Can you work these out from the model? Positions are in its coordinate system, mm. A direction names the side the tool comes from. Coordinates: 2 decimals unless noted, no trailing zeros. Loops run counter-clockwise (first coordinate to the right, second up) from the corner with the lowest first, then second, coordinate; pieces in that order, holes last.
```python
from build123d import *

# Parameters (mm, degrees)
SKETCH_1_W                  = 35
SKETCH_1_H                  = 42
EXTRUDE_1_DEPTH             = 4
SKETCH_2_R                  = 1.5
SKETCH_2_R_2                = 9
CUT_EXTRUDE_1_DEPTH         = 8
SKETCH_3_R                  = 3
CUT_EXTRUDE_2_DEPTH         = 4
HOLE_WIZARD_M4_1_AT_2_COUNT = 2
HOLE_WIZARD_M4_1_AT_2_PITCH = 25
SKETCH_9_R                  = 2
CUT_EXTRUDE_3_DEPTH         = 5.1
CUT_EXTRUDE_4_DEPTH         = 29.482450737
CUT_EXTRUDE_4_DEPTH_BACK    = 29.482450737
SKETCH_10_W                 = 15
SKETCH_10_H                 = 8
SKETCH_10_W_2               = 5
SKETCH_10_H_2               = 20
FILLET_2_R                  = 1
CHAMFER_1_SIZE              = 1


with BuildPart() as part:
    # 草图1 → 凸台-拉伸1 (new, symmetric)
    with BuildSketch(Plane.XY):
        Rectangle(SKETCH_1_W, SKETCH_1_H)
    extrude(amount=EXTRUDE_1_DEPTH, both=True)

    # 草图2 → 切除-拉伸1 (cut)
    with BuildSketch(Plane.XY.offset(4)):
        with Locations((0, 13.5)):
            Circle(SKETCH_2_R)
        with Locations((11.691342951, -6.75)):
            Circle(SKETCH_2_R)
        with Locations((-11.691342951, -6.75)):
            Circle(SKETCH_2_R)
        Circle(SKETCH_2_R_2)
    extrude(amount=-CUT_EXTRUDE_1_DEPTH, mode=Mode.SUBTRACT)

    # 草图3 → 切除-拉伸2 (cut)
    with BuildSketch(Plane.XY.offset(4)):
        with Locations((-11.691342951, -6.75)):
            Circle(SKETCH_3_R)
        with Locations((11.691342951, -6.75)):
            Circle(SKETCH_3_R)
        with Locations((0, 13.5)):
            Circle(SKETCH_3_R)
    extrude(amount=-CUT_EXTRUDE_2_DEPTH, mode=Mode.SUBTRACT)

    # 草图8 → M4 螺纹孔1 (revolve, cut)
    with BuildSketch(Plane(origin=(-12.5, 21, 0), x_dir=(0, 0, 1), z_dir=(1, 0, 0))):
        Polygon((0, 0), (0, 10.991420021), (1.65, 10), (1.65, 0), align=None)
    hole_wizard_m4_1 = revolve(axis=Axis((-12.5, 27.35, 0), (0, -1, 0)), mode=Mode.SUBTRACT)

    # M4 螺纹孔1 at 2: M4 螺纹孔1 ×2
    with Locations(*[(i * HOLE_WIZARD_M4_1_AT_2_PITCH, 0, 0) for i in range(1, HOLE_WIZARD_M4_1_AT_2_COUNT)]):
        add(hole_wizard_m4_1, mode=Mode.SUBTRACT)

    # 镜向1: M4 螺纹孔1 across plane
    add(hole_wizard_m4_1.mirror(Plane.ZX), mode=Mode.SUBTRACT)

    # 镜向1 copy 1 sketch → 镜向1 copy 1 (revolve, cut)
    with BuildSketch(Plane(origin=(12.5, -21, 0), x_dir=(0, 0, 1), z_dir=(1, 0, 0))):
        Polygon((0, 0), (0, -10.991420021), (1.65, -10), (1.65, 0), align=None)
    revolve(axis=Axis((12.5, -27.35, 0), (0, -1, 0)), mode=Mode.SUBTRACT)

    # 草图9 → 切除-拉伸3 (cut)
    with BuildSketch(Plane(origin=(0, 0, -4), x_dir=(-1, 0, 0), z_dir=(0, 0, -1))):
        with Locations((0, -12.15)):
            Circle(SKETCH_9_R)
        with Locations((-10.522208656, 6.075)):
            Circle(SKETCH_9_R)
        with Locations((10.522208656, 6.075)):
            Circle(SKETCH_9_R)
    extrude(amount=-CUT_EXTRUDE_3_DEPTH, mode=Mode.SUBTRACT)

    # 草图10 → 切除-拉伸4 (cut, two sides: drawn at the far end of the back side and taken through both)
    with BuildSketch(Plane(origin=(0, 0, -4), x_dir=(-1, 0, 0), z_dir=(0, 0, -1)).offset(-CUT_EXTRUDE_4_DEPTH_BACK)):
        with Locations((0, 21)):
            Rectangle(SKETCH_10_W, SKETCH_10_H)
        with Locations((0, -21)):
            Rectangle(SKETCH_10_W, SKETCH_10_H)
        with Locations((17.5, 0)):
            Rectangle(SKETCH_10_W_2, SKETCH_10_H_2)
        with Locations((-17.5, 0)):
            Rectangle(SKETCH_10_W_2, SKETCH_10_H_2)
    extrude(amount=CUT_EXTRUDE_4_DEPTH + CUT_EXTRUDE_4_DEPTH_BACK, mode=Mode.SUBTRACT)

    # 圆角2
    fillet_2_edges = [part.edges().sort_by_distance(p)[0] for p in [
        (-7.5, 21, 0),
        (-7.5, 17, 0),
        (7.5, 21, 0),
        (7.5, 17, 0),
        (-7.5, -21, 0),
        (-7.5, -17, 0),
        (7.5, -21, 0),
        (7.5, -17, 0),
        (-17.5, -10, 0),
        (-15, -10, 0),
        (-17.5, 10, 0),
        (-15, 10, 0),
        (15, 10, 0),
        (17.5, -10, 0),
        (15, -10, 0),
        (17.5, 10, 0),
        (17.5, -21, 0),
        (-17.5, -21, 0),
        (-17.5, 21, 0),
        (17.5, 21, 0),
    ]]
    fillet(fillet_2_edges, radius=FILLET_2_R)

    # 倒角1
    chamfer_1_edges = [part.edges().sort_by_distance(p)[0] for p in [
        (-9, 0, -4),
        (-9, 0, 4),
    ]]
    chamfer(chamfer_1_edges, length=CHAMFER_1_SIZE)


solid = part.part
```
Item 1: We'd pull the mould along Y, two halves only. Please class faces 4 (the face through (-14.3, 21, 0.1)), 5 (the face through (10.7, -21, 0.1)), 6 (the face through (-10.08, -4.22, 2.03)), 7 (the face through (0, 12, -2)): +Y half, -Y half, draft (parallel to the pull), parting line (faces both ways), or undercut.
Results are:
face 4: +Y half
face 5: -Y half
face 6: undercut
face 7: undercut
Item 2: Suppose I cut it at A-A, the plane x = 0. Please give me the cut outline in (y, z).
Results are:
outline: (-17, -4) - (-14.15, -4) - (-14.15, 1.1) - (-10.15, 1.1) - (-10.15, -4) - (-10, -4) - (-9, -3) - (-9, 3) - (-10, 4) - (-17, 4) - close; (9, -3) - (10, -4) - (12, -4) - (12, 0) - (10.5, 0) - (10.5, 4) - (10, 4) - (9, 3) - close; (15, -4) - (17, -4) - (17, 4) - (16.5, 4) - (16.5, 0) - (15, 0) - close
Item 3: I need wall thicknesses on line 1 along X through (y, z) = (-18.5, 0); line 2 along Y through (x, z) = (-16, 2); line 3 along X through (y, z) = (-5, 0.5). Which ranges of each line are inside material? Lowest first, please.
Results are:
line 1: x = -17.5 to -14.15, -10.85 to -7.5, 7.5 to 10.85, 14.15 to 17.5
line 2: y = -21 to -10, 10 to 21
line 3: x = -15 to -14.13, -9.25 to -7.48, 7.48 to 9.25, 14.13 to 15
Item 4: Suppose I cut it at B-B, the plane y = -12.15. Please give me the cut outline in (x, z), plus the area to 3 significant figures.
Results are:
outline: (-17.5, -4) - (-2, -4) - (-2, 1.1) - (2, 1.1) - (2, -4) - (17.5, -4) - (17.5, 4) - (-17.5, 4) - close; hole circle Ø3.3 at (-12.5, 0); hole circle Ø3.3 at (12.5, 0)
area: 242 mm2
Item 5: On a 3-axis mill with a long thin cutter (end or side, diameter ignored), from which of +Z, -Z, +X, -X, +Y, -Y can I reach the whole of each face in a straight line? I mean faces 1 (the face through (17.199, -10.285, 0.056)), 2 (the face through (0, -12, 1.1)), 3 (the face through (-7.801, 20.715, 0.056)). Say none if no direction works.
Results are:
face 1: +Z, -Z, +X
face 2: -Z
face 3: +Z, -Z, +Y
Item 6: I'm going to push flat-ended pins straight in: P1, Ø6, axis at x = -2.5, y = -6.5, coming from the +Z side; P2, Ø2.5, axis at x = 10.52, y = 6.08, coming from the -Z side; P3, Ø4.5, axis at x = 12.5, z = 0, coming from the +Y side; P4, Ø5, axis at x = 2.5, y = 3.5, coming from the +Z side. Where does each tip first touch, or does it pass through?
Results are:
P1: stops at z = 3.96
P2: stops at z = 1.1
P3: stops at y = 21
P4: passes through
